Source: CAD feature listing. Evaluate the final solid. Frame: model axes, mm. Face numbers are marked on the shaded views. Give positions to 0.01 mm unless a question says otherwise; leave off trailing zeros. Loops run counter-clockwise (first coordinate to the right, second up) from the corner with the lowest first, then second, coordinate; pieces in that order, holes last. Notation, with made-up numbers: (10, 19.25) -> (32, 19.25) arc R28 ccw to (32, 51.25) -> close; hole circle Ø11 at (-20, -16.75). An arc over 180 degrees is marked (long way). Return JSON: item names as keys, results as strings. Group by question number.
(1) Cut plane A-A on y = 0. Return loops of the section in (x, z), then the cut area to 3 significant figures.
(2) Pin query (flat end, axial travel): pin 1 (4 mm diameter, centred on x = 0, y = 0, fed in from +Z) (3 decimals). Return the tip coordinate at first contact, or that it passes through.
(3) Ray query, line 1 (Y direction, x = 3.25, z = 0); line 2 (Y direction, x = 1, z = 4.5). Return the intervals inside material, ascending. Write a range as from..to.
(4) Cut plane B-B on z = -6.5. Return loops of the section in (x, y).
(5) Draft query along Y for the marked faces 1, 2, 3 and 4. Return one class per face: released by +Y, released by -Y, zero draft, split by the parting line, or undercut.
(6) Cut plane C-C on z = 1.25. Return loops of the section in (x, y), then the cut area to 3 significant figures.
```python
from build123d import *

# Parameters (mm, degrees)
SKETCH1_W           = 19
SKETCH1_H           = 19
BOSS_EXTRUDE1_DEPTH = 9.5
SKETCH2_R           = 2.5
CUT_EXTRUDE1_DEPTH  = 25
SKETCH3_R           = 2.5
CUT_EXTRUDE2_DEPTH  = 25


with BuildPart() as part:
    # Sketch1 → Boss-Extrude1 (new body, symmetric)
    with BuildSketch(Plane.XY):
        Rectangle(SKETCH1_W, SKETCH1_H)
    extrude(amount=BOSS_EXTRUDE1_DEPTH, both=True)

    # Sketch2 → Cut-Extrude1 (cut)
    with BuildSketch(Plane.XY.offset(9.5)):
        Circle(SKETCH2_R)
    extrude(amount=-CUT_EXTRUDE1_DEPTH, mode=Mode.SUBTRACT)

    # Sketch3 → Cut-Extrude2 (cut)
    with BuildSketch(Plane(origin=(9.5, 0, 0), x_dir=(0, 0, -1), z_dir=(1, 0, 0))):
        Circle(SKETCH3_R)
    extrude(amount=-CUT_EXTRUDE2_DEPTH, mode=Mode.SUBTRACT)


solid = part.part
```
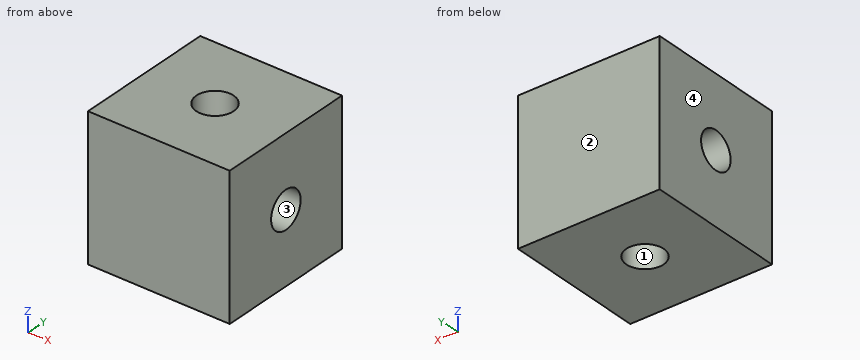
Answers:
{
 "1": {"outline": "(-9.5, -9.5) -> (-2.5, -9.5) -> (-2.5, -2.5) -> (-9.5, -2.5) -> close; (-9.5, 2.5) -> (-2.5, 2.5) -> (-2.5, 9.5) -> (-9.5, 9.5) -> close; (2.5, -9.5) -> (9.5, -9.5) -> (9.5, -2.5) -> (2.5, -2.5) -> close; (2.5, 2.5) -> (9.5, 2.5) -> (9.5, 9.5) -> (2.5, 9.5) -> close", "area": "196 mm²"},
 "2": {"pin 1": "through"},
 "3": {"line 1": "-9.5..-2.5, 2.5..9.5", "line 2": "-9.5..-2.29, 2.29..9.5"},
 "4": {"outline": "(-9.5, -9.5) -> (9.5, -9.5) -> (9.5, 9.5) -> (-9.5, 9.5) -> close; hole circle Ø5 at (0, 0)"},
 "5": {"face 1": "undercut", "face 2": "released by +Y", "face 3": "undercut", "face 4": "zero draft"},
 "6": {"outline": "(-9.5, -9.5) -> (9.5, -9.5) -> (9.5, -2.17) -> (1.25, -2.17) arc R2.5 cw to (-1.25, -2.17) -> (-9.5, -2.17) -> close; (-9.5, 2.17) -> (-1.25, 2.17) arc R2.5 cw to (1.25, 2.17) -> (9.5, 2.17) -> (9.5, 9.5) -> (-9.5, 9.5) -> close", "area": "278 mm²"}
}
